Verification items for the finished model (mm, model axes). Face numbers are marked on the shaded views. A direction names the side the tool comes from. Give positions to 0.01 mm unless a question says otherwise; leave off trailing zeros. Write each loop counter-clockwise with the first axis right and the second up, starting at its lowest first coordinate (ties: lowest second). Pieces come first, ordered by that corner, then holes. Notation, with made-up numbers: (56, 55.5) - (62, 55.5) arc R31 cw to (62, 82.5) - close; hole circle Ø3 at (-35.5, -2.5). An arc over 180 degrees is marked (long way). Answer as a JSON object with one key per item and string values. Group by question number.
Item 1: Tool access check on the marked faces 4 and 5. Record the directions out of +Z, -Z, +X, -X, +Y, -Y that give a thin tool (end or side, any length) a straight path to the whole face; none if there is none.
Item 2: Go/stop test with flat-tipped pins: pin 1 (2.5 mm diameter, centred on x = 6.75, y = 11.69, fed in from +Z); pin 2 (1.8 mm diameter, centred on x = -4.5, z = 2.5, fed in from -Y); pin 3 (1 mm diameter, centred on x = -1.5, y = 0.5, fed in from -Z); pin 4 (3 mm diameter, centred on x = -13.5, y = 0, fed in from +Z). Record where each tip stops, or that it passes through.
Item 3: Sectioned sample at B-B, the plane z = 4.5. Count the separate pieces of the cut face and the enclosed holes in it, and give its area (3 significant figures).
Item 4: Sectioned sample at C-C, the plane y = 6. Record the boundary of the cut face in (x, z), and give its area (3 significant figures).
Item 5: Scan lines: line 1 along Y through (x, z) = (-7, 1.5); line 2 along X through (y, z) = (-11, 4.75); line 3 along X through (y, z) = (-0.5, 3.5). Record each from-to range of solid material in increasing order. Write a range as [from, to].
Item 6: Draft check along X on the marked faces 1, 2 and 3. Enter one of: +X half, -X half, draft (parallel to the pull), parting line (faces both ways), or undercut.
Item 7: Sectioned sample at A-A, the plane x = 13.5. Record the boundary of the cut face in (y, z).
```python
from build123d import *

# Parameters (mm, degrees)
BOSS_EXTRUDE1_DEPTH  = 9.6
CHAMFER2_SIZE        = 0.6
CUT_EXTRUDE2_DEPTH   = 2.5
M2_CLEARANCE_HOLE1_D = 2.6
CUT_EXTRUDE3_START   = -9.6
CUT_EXTRUDE3_DEPTH   = 5.5
CHAMFER3_SIZE        = 1.5


with BuildPart() as part:
    # Sketch1 → Boss-Extrude1 (new body)
    with BuildSketch(Plane.XY):
        with BuildLine():
            ThreePointArc((-11.756599923, -15.949743136), (-6.144180323, -14.833363466), (-2.965, -19.591343059))
            Line((-2.965, -19.591343059), (2.965, -19.591343059))
            ThreePointArc((2.965, -19.591343059), (6.144180323, -14.833363466), (11.756599923, -15.949743136))
            Line((11.756599923, -15.949743136), (15.949743136, -11.756599923))
            ThreePointArc((15.949743136, -11.756599923), (14.833363466, -6.144180323), (19.591343059, -2.965))
            Line((19.591343059, -2.965), (19.591343059, 2.965))
            ThreePointArc((19.591343059, 2.965), (14.833363466, 6.144180323), (15.949743136, 11.756599923))
            Line((15.949743136, 11.756599923), (11.756599923, 15.949743136))
            ThreePointArc((11.756599923, 15.949743136), (6.144180323, 14.833363466), (2.965, 19.591343059))
            Line((2.965, 19.591343059), (-2.965, 19.591343059))
            ThreePointArc((-2.965, 19.591343059), (-6.144180323, 14.833363466), (-11.756599923, 15.949743136))
            Line((-11.756599923, 15.949743136), (-15.949743136, 11.756599923))
            ThreePointArc((-15.949743136, 11.756599923), (-14.833363466, 6.144180323), (-19.591343059, 2.965))
            Line((-19.591343059, 2.965), (-19.591343059, -2.965))
            ThreePointArc((-19.591343059, -2.965), (-14.833363466, -6.144180323), (-15.949743136, -11.756599923))
            Line((-15.949743136, -11.756599923), (-11.756599923, -15.949743136))
        make_face()
    extrude(amount=BOSS_EXTRUDE1_DEPTH)

    # Chamfer2
    chamfer2_edges = [part.edges().sort_by_distance(p)[0] for p in [
        (-19.591343059, 0, 9.6),
        (-13.853171529, 13.853171529, 0),
        (0, 19.591343059, 0),
        (13.853171529, 13.853171529, 0),
        (19.591343059, 0, 0),
        (-13.853171529, -13.853171529, 9.6),
        (13.853171529, -13.853171529, 0),
        (0, -19.591343059, 0),
        (-13.853171529, -13.853171529, 0),
        (-19.591343059, 0, 0),
        (0, -19.591343059, 9.6),
        (13.853171529, -13.853171529, 9.6),
        (19.591343059, 0, 9.6),
        (13.853171529, 13.853171529, 9.6),
        (0, 19.591343059, 9.6),
        (-13.853171529, 13.853171529, 9.6),
    ]]
    chamfer(chamfer2_edges, length=CHAMFER2_SIZE)

    # Sketch4 → Cut-Extrude2 (cut)
    with BuildSketch(Plane.XY.offset(9.6)):
        with BuildLine():
            ThreePointArc((14.441692106, -1.95061736), (16, 0), (14.441692106, 1.95061736))
            Line((14.441692106, 1.95061736), (6.69085075, 3.70569527))
            Line((6.69085075, 3.70569527), (6.495190528, 3.75))
            Line((6.495190528, 3.75), (6.554651618, 3.941599088))
            Line((6.554651618, 3.941599088), (6.750311839, 3.897294358))
            Line((6.750311839, 3.897294358), (9.101143263, 11.472284348))
            ThreePointArc((9.101143263, 11.472284348), (8.1, 14.029611541), (5.384718053, 13.617963443))
            Line((5.384718053, 13.617963443), (0, 7.794588715))
            Line((0, 7.794588715), (-5.384718053, 13.617963443))
            ThreePointArc((-5.384718053, 13.617963443), (-8.1, 14.029611541), (-9.101143263, 11.472284348))
            Line((-9.101143263, 11.472284348), (-6.750311839, 3.897294358))
            Line((-6.750311839, 3.897294358), (-14.485861316, 2.145679096))
            ThreePointArc((-14.485861316, 2.145679096), (-16.2, 0), (-14.485861316, -2.145679096))
            Line((-14.485861316, -2.145679096), (-6.750311839, -3.897294358))
            Line((-6.750311839, -3.897294358), (-9.101143263, -11.472284348))
            ThreePointArc((-9.101143263, -11.472284348), (-8.1, -14.029611541), (-5.384718053, -13.617963443))
            Line((-5.384718053, -13.617963443), (0, -7.794588715))
            Line((0, -7.794588715), (5.384718053, -13.617963443))
            ThreePointArc((5.384718053, -13.617963443), (8.1, -14.029611541), (9.101143263, -11.472284348))
            Line((9.101143263, -11.472284348), (6.750311839, -3.897294358))
            Line((6.750311839, -3.897294358), (6.554651618, -3.941599088))
            Line((6.554651618, -3.941599088), (6.495190528, -3.75))
            Line((6.495190528, -3.75), (6.69085075, -3.70569527))
            Line((6.69085075, -3.70569527), (14.441692106, -1.95061736))
        make_face()
    extrude(amount=-CUT_EXTRUDE2_DEPTH, mode=Mode.SUBTRACT)

    # M2 Clearance Hole1 (through all)
    with Locations(Plane.XY.offset(7.1)):
        with Locations((13.5, 0), (6.75, -11.691342951), (-6.75, -11.691342951), (-13.5, 0), (-6.75, 11.691342951), (6.75, 11.691342951)):
            Hole(M2_CLEARANCE_HOLE1_D / 2)

    # Sketch3<2> → Cut-Extrude3 (cut)
    with BuildSketch(Plane.XY.offset(9.6).offset(CUT_EXTRUDE3_START)):
        with BuildLine():
            Line((-2, -1.5), (-5.5, -1.5))
            Line((-5.5, -1.5), (-5.5, 1.5))
            Line((-5.5, 1.5), (-2, 1.5))
            ThreePointArc((-2, 1.5), (0, 2.5), (2, 1.5))
            Line((2, 1.5), (5.5, 1.5))
            Line((5.5, 1.5), (5.5, -1.5))
            Line((5.5, -1.5), (2, -1.5))
            ThreePointArc((2, -1.5), (0, -2.5), (-2, -1.5))
        make_face()
    extrude(amount=CUT_EXTRUDE3_DEPTH, mode=Mode.SUBTRACT)

    # Chamfer3
    chamfer3_edges = [part.edges().sort_by_distance(p)[0] for p in [
        (-3.75, -1.5, 5.5),
        (0, -2.5, 5.5),
        (3.75, -1.5, 5.5),
        (5.5, 0, 5.5),
        (3.75, 1.5, 5.5),
        (0, 2.5, 5.5),
        (-3.75, 1.5, 5.5),
        (-5.5, 0, 5.5),
    ]]
    chamfer(chamfer3_edges, length=CHAMFER3_SIZE - 0.0001)  # a hair under: the kernel refuses the full size


solid = part.part
```
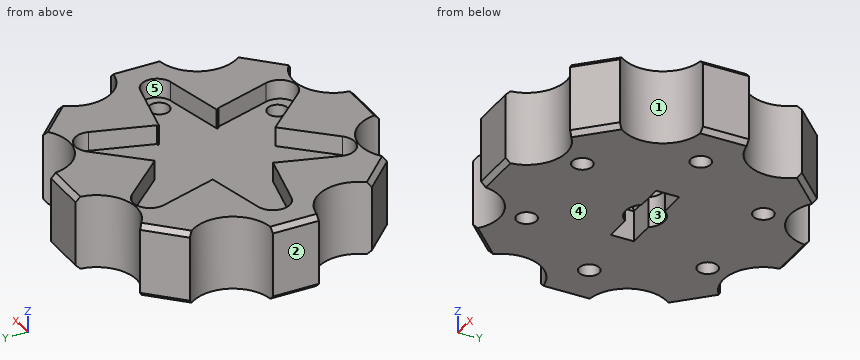
Geometry check:
{
 "1": {"face 4": "-Z, +X, -X, +Y, -Y", "face 5": "+Z"},
 "2": {"pin 1": "through", "pin 2": "y = -17.11", "pin 3": "z = 4.54", "pin 4": "z = 7.1"},
 "3": {"separate pieces": "1", "enclosed holes": "7", "area": "965 mm^2"},
 "4": {"outline": "(-14.9, 0) - (14.9, 0) - (14.9, 9.6) - (7.4, 9.6) - (7.4, 7.1) - (-7.4, 7.1) - (-7.4, 9.6) - (-14.9, 9.6) - close", "area": "249 mm^2"},
 "5": {"line 1": "[-14.56, -12.97], [-10.42, 10.42], [12.97, 14.56]", "line 2": "[-15.33, -7.85], [-5.65, 5.65], [7.85, 15.33]", "line 3": "[-19.59, -14.7], [-12.3, -5.5], [5.5, 12.3], [14.7, 19.59]"},
 "6": {"face 1": "+X half", "face 2": "-X half", "face 3": "undercut"},
 "7": {"outline": "(-14.21, 0.6) - (-13.36, 0) - (-1.3, 0) - (-1.3, 7.1) - (-2.16, 7.1) - (-2.16, 9.6) - (-13.36, 9.6) - (-14.21, 9) - close; (1.3, 0) - (13.36, 0) - (14.21, 0.6) - (14.21, 9) - (13.36, 9.6) - (2.16, 9.6) - (2.16, 7.1) - (1.3, 7.1) - close"}
}
